Design review of the part built by this model. Coordinates are the model's own, in mm. A direction names the side the tool comes from. Give positions to 0.01 mm unless a question says otherwise; leave off trailing zeros. Loops run counter-clockwise (first coordinate to the right, second up) from the corner with the lowest first, then second, coordinate; pieces in that order, holes last. Notation, with made-up numbers: M 30.5,10.5 L 39.5,10.5 A29 ccw 39.5,36.5 Z; hole C -6,70.5 d7. An arc over 180 degrees is marked long. Answer as CSV lines item,"result".
```python
from build123d import *


with BuildPart() as f1:
    # F0 (on Front) → F1 (revolve)
    with BuildSketch(Plane.XZ):
        with BuildLine():
            Line((11.530839, 36.909778), (8.377308, 48.545218))
            Line((8.377308, 48.545218), (7.237623, 48.545218))
            Line((7.237623, 48.545218), (10.469142, 36.622028))
            ThreePointArc((10.469142, 36.622028), (10.644584, 33.299521), (9.438111, 30.198835))
            Line((9.438111, 30.198835), (0.794426, 22.659409))
            ThreePointArc((0.794426, 22.659409), (0.424202, 22.438515), (0, 22.361623))
            Line((0, 22.361623), (0, 0.875514))
            Line((0, 0.875514), (8.827639, 0.875514))
            Line((8.827639, 0.875514), (8.827639, 1.66595))
            Line((8.827639, 1.66595), (4.268712, 1.817272))
            ThreePointArc((4.268712, 1.817272), (1.867439, 2.882665), (0.882294, 5.317959))
            Line((0.882294, 5.317959), (0.882294, 20.650616))
            ThreePointArc((0.882294, 20.650616), (1.191417, 21.38592), (1.706291, 21.995127))
            Line((1.706291, 21.995127), (10.27026, 29.465022))
            ThreePointArc((10.27026, 29.465022), (11.718112, 33.048966), (11.530839, 36.909778))
        make_face()
    revolve(axis=Axis((0, 0, 23.284463), (0, 0, -1)))


solid = f1.part
```
1. We need section B-B, the plane z = 24.5. Write out the cut boundary in (x, y), plus the area to 3 significant figures.
Answer block:
outline,"C 0,0 d9.16; hole C 0,0 d5.81"
area,"39.3 mm²"
2. We need section C-C, the plane z = 4.5. Write out the cut boundary in (x, y).
Answer block:
outline,"C 0,0 d1.96"
3. We need section A-A, the plane z = 13. Write out the cut boundary in (x, y), plus the area to 3 significant figures.
Answer block:
outline,"C 0,0 d1.76"
area,"2.45 mm²"
4. To check wall thickness, follow L1, parallel to Y at x = -3.25, z = 37; L2, parallel to Y at x = -7, z = 39.5; L3, parallel to X at y = 5, z = 38. State the ranges of each line that lie inside material, in increasing order. Write a range as [from, to].
Answer block:
L1,"[-11.04, -9.84], [9.84, 11.04]"
L2,"[-8.26, -6.7], [6.7, 8.26]"
L3,"[-10.06, -8.77], [8.77, 10.06]"
5. For faces 1 (the cylindrical face through (0.474, -0.744, 13.092)), 2 (the flat face through (-3, -7, 48.545)), list the 3-axis set-ups (+Z, -Z, +X, -X, +Y, -Y) from which the entire face can be reached by the end or side of a thin tool; tool diameter is ignored.
Answer block:
face 1,"none"
face 2,"+Z, +X, -X, +Y, -Y"
6. The part is to be moulded in two halves that separate along X. For faces 3 (the flat face through (0, 0, 0.876)), 4 (the cylindrical face through (8.42, -2.65, 1.28)), 5 (the conical face through (-1.06, -8.09, 45.15)), say which applies: pulls with the +X half, pulls with the -X half, needs draft (parallel to the pull), parting line crosses it, or undercut.
Answer block:
face 3,"needs draft"
face 4,"parting line crosses it"
face 5,"undercut"
7. For P1, Ø5, axis at x = -9.5, y = -4, coming from the +Z side; P2, Ø3, axis at x = 9, z = 25.5, coming from the +Y side; P3, Ø1.5, axis at x = 6.5, z = 34.5, coming from the -Y side, all flat-tipped, find the tip position at first contact; note any pin that passes through.
Answer block:
P1,"z = 48.55"
P2,"through"
P3,"y = -10.36"
